Source: CAD feature listing. Evaluate the final solid. Frame: model axes, mm. A direction names the side the tool comes from. Coordinates: 2 decimals unless noted, no trailing zeros. Write each loop counter-clockwise with the first axis right and the second up, starting at its lowest first coordinate (ties: lowest second). Pieces come first, ordered by that corner, then holes. Notation, with made-up numbers: M 82.25,-39 L 103.25,-39 A17 ccw 103.25,-33 Z; hole C 6.25,86.5 d9. An arc over 180 degrees is marked long. One line per item, written item: value. Start each with the question number.
Item 1: Pin query (flat end, axial travel): P1, Ø10, axis at x = -7.5, y = -6, coming from the +Z side; P2, Ø1, axis at x = 1.5, y = 10.5, coming from the +Z side; P3, Ø4, axis at x = -9.5, z = 7, coming from the -Y side. Return the tip coordinate at first contact, or that it passes through.
Item 2: Cut plane C-C, the plane z = 7.25. Output: boundary loops of the cut face in (x, y).
Item 3: Set-up query: faces 1 (the flat face through (10, 0, 8)), 2 (the cylindrical face through (-12.248, 0.099, 4.958)). Return all of +Z, -Z, +X, -X, +Y, -Y with unobstructed straight access to the full face (end or side cutting, diameter ignored); none if empty.
Item 4: Ray query, L1, parallel to Z at x = -1.5, y = -16.5; L2, parallel to X at y = -2, z = 6.25; L3, parallel to Y at x = -4, z = 1.75. Return the intervals inside material, ascending. Write a range as from..to.
Item 5: Mould query, pull axis X, two halves, no side actions, for faces 3 (the cylindrical face through (0.21, 41.43, 0.6)), 4 (the cylindrical face through (-14.43, 0.59, 0.6)), 5 (the cylindrical face through (12.248, -0.099, 4.958)). Classes: released by +X, released by -X, zero draft, split by the parting line, or undercut.
```python
from build123d import *

# Parameters (mm, degrees)
SKETCH1_W           = 30
SKETCH1_H           = 84
SKETCH1_R           = 2.25
BOSS_EXTRUDE1_DEPTH = 2
SKETCH1_4_R         = 2.25
BOSS_EXTRUDE2_DEPTH = 8
FILLET1_R           = 2


with BuildPart() as part:
    # Sketch1 → Boss-Extrude1 (new body)
    with BuildSketch(Plane.XY):
        Rectangle(SKETCH1_W, SKETCH1_H)
        with Locations((-10, 0)):
            Circle(SKETCH1_R, mode=Mode.SUBTRACT)
        with Locations(Location((10, 0, 0), (0, 0, 180))):
            Circle(SKETCH1_R, mode=Mode.SUBTRACT)
    extrude(amount=BOSS_EXTRUDE1_DEPTH)

    # Sketch1<4> → Boss-Extrude2 (add)
    with BuildSketch(Plane.XY):
        with Locations((-10, 0)):
            Circle(SKETCH1_4_R)
        with Locations(Location((10, 0, 0), (0, 0, 180))):
            Circle(SKETCH1_4_R)
    extrude(amount=BOSS_EXTRUDE2_DEPTH)

    # Fillet1
    fillet1_edges = [part.edges().sort_by_distance(p)[0] for p in [
        (0, 42, 0),
        (-15, 0, 0),
        (0, -42, 0),
        (15, 0, 0),
    ]]
    fillet(fillet1_edges, radius=FILLET1_R - 0.0001)  # a hair under: the kernel refuses the full size


solid = part.part
```
From the geometry:
1. P1: stops at z = 8
1. P2: stops at z = 2
1. P3: stops at y = -2.25
2. outline: C -10,0 d4.5; C 10,0 d4.5
3. face 1: +Z, +X, -X, +Y, -Y
3. face 2: +Z
4. L1: z = 0..2
4. L2: x = -11.03..-8.97, 8.97..11.03
4. L3: y = -41.98..41.98
5. face 3: zero draft
5. face 4: released by -X
5. face 5: undercut
